Part model, mm, in its own coordinate system. Face numbers are marked on the shaded views. A direction names the side the tool comes from. Coordinates: 2 decimals unless noted, no trailing zeros. Loops run counter-clockwise (first coordinate to the right, second up) from the corner with the lowest first, then second, coordinate; pieces in that order, holes last. Notation, with made-up numbers: (61, 76) - (116, 76) arc R16 cw to (116, 98) - close; hole circle Ø8 at (65, 29.5). An arc over 180 degrees is marked (long way). Answer as CSV lines item,"result".
from build123d import *

# Parameters (mm, degrees)
SKETCH_1_W                = 60
SKETCH_1_H                = 60
EXTRUDE_1_DEPTH           = 12.6
CHAMFER_1_SIZE            = 2
SKETCH_2_W                = 35
SKETCH_2_H                = 35
EXTRUDE_2_DEPTH           = 0.4
FILLET_1_R                = 2
HOLE_WIZARD_1_D           = 3.4
HOLE_WIZARD_1_CBORE_D     = 6
HOLE_WIZARD_1_CBORE_DEPTH = 5
HOLE_WIZARD_M3_1_D        = 2.5
HOLE_WIZARD_M3_1_DEPTH    = 3.5
HOLE_WIZARD_M3_1_TIP      = 0.751075774
SKETCH_7_R                = 2.5
EXTRUDE_3_DEPTH           = 10


with BuildPart() as part:
    # 草图1 → 凸台-拉伸1 (new body)
    with BuildSketch(Plane.XY):
        Rectangle(SKETCH_1_W, SKETCH_1_H)
    extrude(amount=EXTRUDE_1_DEPTH)

    # 倒角1
    chamfer_1_edges = [part.edges().sort_by_distance(p)[0] for p in [
        (30, -30, 6.3),
        (-30, -30, 6.3),
        (-30, 30, 6.3),
        (30, 30, 6.3),
    ]]
    chamfer(chamfer_1_edges, length=CHAMFER_1_SIZE)

    # 草图2 → 凸台-拉伸2 (add)
    with BuildSketch(Plane.XY.offset(12.6)):
        Rectangle(SKETCH_2_W, SKETCH_2_H)
    extrude(amount=EXTRUDE_2_DEPTH)

    # 圆角1
    fillet_1_edges = [part.edges().sort_by_distance(p)[0] for p in [
        (17.5, -17.5, 12.8),
        (17.5, 17.5, 12.8),
        (-17.5, 17.5, 12.8),
        (-17.5, -17.5, 12.8),
    ]]
    fillet(fillet_1_edges, radius=FILLET_1_R)

    # 孔1 (through all)
    with Locations(Plane(origin=(-25, 25, 12.6), x_dir=(1, 0, 0), z_dir=(0, 0, 1))):
        with Locations((0, 0), (50, 0), (0, -50), (50, -50)):
            CounterBoreHole(HOLE_WIZARD_1_D / 2, HOLE_WIZARD_1_CBORE_D / 2, HOLE_WIZARD_1_CBORE_DEPTH)

    # M3 螺纹孔1
    with Locations(Plane(origin=(-12.5, 12.5, 13), x_dir=(1, 0, 0), z_dir=(0, 0, 1))):
        with Locations((0, 0), (25, 0), (25, -25), (0, -25)):
            Hole(HOLE_WIZARD_M3_1_D / 2, depth=HOLE_WIZARD_M3_1_DEPTH)
            with Locations((0, 0, -(HOLE_WIZARD_M3_1_DEPTH + HOLE_WIZARD_M3_1_TIP / 2))):  # 118° drill point
                Cone(0, HOLE_WIZARD_M3_1_D / 2, HOLE_WIZARD_M3_1_TIP, mode=Mode.SUBTRACT)

    # 草图7 → 凸台-拉伸3 (add)
    with BuildSketch(Plane.XZ.offset(30)):
        with Locations((-18.5, 5)):
            Circle(SKETCH_7_R)
    extrude(amount=EXTRUDE_3_DEPTH)


solid = part.part
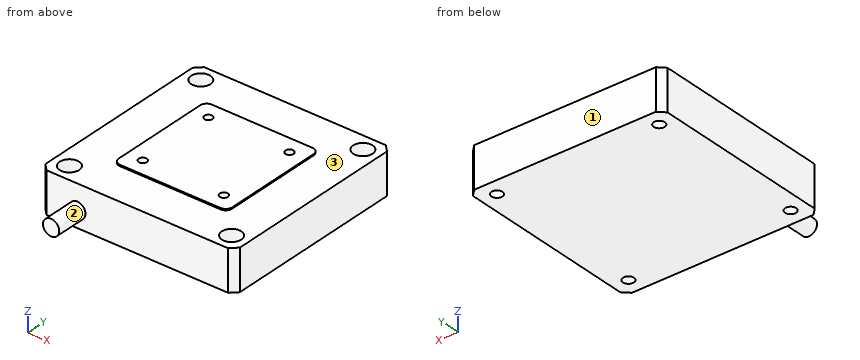
Q1. Saw through at D-D (z = 5). Give the cut face in (x, y).
Results:
outline,"(-30, -28) - (-28, -30) - (-21, -30) - (-21, -40) - (-16, -40) - (-16, -30) - (28, -30) - (30, -28) - (30, 28) - (28, 30) - (-28, 30) - (-30, 28) - close; hole circle Ø3.4 at (-25, -25); hole circle Ø3.4 at (-25, 25); hole circle Ø3.4 at (25, -25); hole circle Ø3.4 at (25, 25)"
Q2. Flat gauge pins, fed straight in: pin 1 (5 mm diameter, centred on x = -26, y = 24.5, fed in from +Z); pin 2 (5.5 mm diameter, centred on x = 25, y = -25, fed in from +Z); pin 3 (4 mm diameter, centred on x = 18.5, z = 6, fed in from -Y). Where does each tip first touch, or does it go through?
Results:
pin 1,"stops at z = 12.6"
pin 2,"stops at z = 7.6"
pin 3,"stops at y = -30"
Q3. Which spindle directions (+Z, -Z, +X, -X, +Y, -Y) get a long thin tool onto all of the face, cutting with end or side? Do the marked faces 1, 2 and 3. Say none if no direction does.
Results:
face 1,"+Z, -Z, +X, -X, +Y"
face 2,"-Y"
face 3,"+Z"
Q4. Saw through at B-B (z = 10.5). Count the separate pieces of the cut face and the enclosed holes in it, then the cut area to 3 significant figures.
Results:
separate pieces,"1"
enclosed holes,"8"
area,"3,460 mm^2"
Q5. Wall check: L1, parallel to Y at x = -25, z = 11.1; L2, parallel to X at y = -12.5, z = 10.6. Give the ranges that are in metal, low to high.
Results:
L1,"y = -30 to -28, -22 to 22, 28 to 30"
L2,"x = -30 to -13.75, -11.25 to 11.25, 13.75 to 30"
Q6. Saw through at A-A (x = 25). Give the cut face in (y, z), then the cut area to 3 significant figures.
Results:
outline,"(-30, 0) - (-26.7, 0) - (-26.7, 7.6) - (-28, 7.6) - (-28, 12.6) - (-30, 12.6) - close; (-23.3, 0) - (23.3, 0) - (23.3, 7.6) - (22, 7.6) - (22, 12.6) - (-22, 12.6) - (-22, 7.6) - (-23.3, 7.6) - close; (26.7, 0) - (30, 0) - (30, 12.6) - (28, 12.6) - (28, 7.6) - (26.7, 7.6) - close"
area,"644 mm^2"
